from build123d import *

# Parameters (mm, degrees)
F0_W        = 50.8
F0_H        = 127
F0_R        = 50.8
F1_DEPTH    = 76.2
F2_T1_DEPTH = 76.2
F3_R        = 63.5


# Not quite as in the source:
# - a fillet or chamfer that OpenCascade refuses, or shapes differently, is made with other operations: its cross-section is extruded or revolved along the edge and cut away or added
# - a feature names something its author has since deleted; it is built from what else it names


with BuildPart() as f1:
    # F0 (on Top) → F1 (new body)
    with BuildSketch(Plane.XY):
        with BuildLine():
            Line((-3842.1031233725, -492.1847614173), (-3653.1472320591, -467.9789534788))
            ThreePointArc((-3653.1472320591, -467.9789534788), (-3683, 0), (-3653.1472320591, 467.9789534788))
            Line((-3653.1472320591, 467.9789534788), (-3842.1031233725, 492.1847614173))
            ThreePointArc((-3842.1031233725, 492.1847614173), (-3873.5, 0), (-3842.1031233725, -492.1847614173))
        make_face()
        Polygon((-3672.3184884479, -419.8900563283), (-3722.8813354916, -424.7929635108), (-3735.1386034477, -298.3858459017), (-3684.5757564041, -293.4829387192), align=None, mode=Mode.SUBTRACT)
        Polygon((-3688.3163611044, -241.9776031163), (-3739.0570382274, -244.4319227962), (-3745.1928374272, -117.5802299885), (-3694.4521603041, -115.1259103086), align=None, mode=Mode.SUBTRACT)
        with Locations((-3721.1, 0)):
            Rectangle(F0_W, F0_H, mode=Mode.SUBTRACT)
        Polygon((-3694.4521603041, 115.1259103086), (-3745.1928374272, 117.5802299885), (-3739.0570382274, 244.4319227962), (-3688.3163611044, 241.9776031163), align=None, mode=Mode.SUBTRACT)
        Polygon((-3684.5757564041, 293.4829387192), (-3735.1386034477, 298.3858459017), (-3722.8813354916, 424.7929635108), (-3672.3184884479, 419.8900563283), align=None, mode=Mode.SUBTRACT)
        with BuildLine():
            Line((-3653.1472320591, -467.9789534788), (-3275.2354494323, -419.5673376017))
            ThreePointArc((-3275.2354494323, -419.5673376016), (-3302, 0), (-3275.2354494323, 419.5673376016))
            Line((-3275.2354494323, 419.5673376017), (-3653.1472320591, 467.9789534788))
            ThreePointArc((-3653.1472320591, 467.9789534788), (-3683, 0), (-3653.1472320591, -467.9789534788))
        make_face()
        with Locations((-3492.5, 0)):
            Circle(F0_R, mode=Mode.SUBTRACT)
        with BuildLine():
            Line((-3627.8456416998, -635), (-3240.367108832, -635))
            ThreePointArc((-3240.367108832, -635), (-3259.5815655268, -527.5718128161), (-3275.2354494323, -419.5673376016))
            Line((-3275.2354494323, -419.5673376017), (-3653.1472320591, -467.9789534788))
            ThreePointArc((-3653.1472320591, -467.9789534788), (-3641.4541483351, -551.6345579938), (-3627.8456416998, -635))
        make_face()
        with BuildLine():
            Line((-3517.3268486167, -1092.2), (-3116.1359341338, -1092.2))
            ThreePointArc((-3116.1359341338, -1092.2000000001), (-3186.4620967161, -865.8309917021), (-3240.367108832, -635))
            Line((-3240.367108832, -635), (-3627.8456416998, -635))
            ThreePointArc((-3627.8456416998, -635), (-3579.8925178131, -865.3661426853), (-3517.3268486167, -1092.1999999999))
        make_face()
        with Locations((-3384.0436300379, -863.6)):
            Circle(F0_R, mode=Mode.SUBTRACT)
    extrude(amount=F1_DEPTH)

    # F2: fillet of radius 762 on 1 edges, made by hand

    # F2_s2 → F2_t1 (join)
    with BuildSketch(Plane.XY):
        with BuildLine():
            ThreePointArc((-3842.1031233725, -492.1847614173), (-3670.9916584142, -676.9720156234), (-3569.4589749529, -907.4423541626))
            Line((-3569.4589749529, -907.4423541626), (-3554.6887998841, -903.6874202833))
            ThreePointArc((-3554.6887998841, -903.6874202833), (-3603.0108161093, -686.1315301017), (-3638.030760754, -466.0424888437))
            Line((-3638.030760754, -466.0424888437), (-3655.0836966942, -452.8624821737))
            ThreePointArc((-3655.0836966942, -452.8624821737), (-3749.5616423509, -464.965386143), (-3832.7858312721, -480.1246756831))
            Line((-3832.7858312721, -480.1246756831), (-3842.1031233725, -492.1847614173))
        make_face()
    extrude(amount=F2_T1_DEPTH)

    # F3
    f3_edges = [f1.edges().sort_by_distance(p)[0] for p in [
        (-3842.103123, -492.184761, 38.1),
        (-3842.103123, 492.184761, 38.1),
        (-3275.235449, 419.567338, 38.1),
        (-3116.135934, -1092.2, 38.1),
        (-3517.326849, -1092.2, 38.1),
    ]]
    fillet(f3_edges, radius=F3_R)


solid = f1.part
Here's how the part is built. I have some questions about the finished solid (model axes, mm). A direction names the side the tool comes from. Round coordinates to 2 decimals unless told otherwise and drop trailing zeros. Loops run counter-clockwise (first coordinate to the right, second up) from the corner with the lowest first, then second, coordinate; pieces in that order, holes last.
1. We'd pull the mould along Y, two halves only. Please class faces 1 (the face through (-3153.62, -1066.79, 38.63)), 2 (the face through (-3666.08, -684.55, 37.57)), 3 (the face through (-3746.5, -1, 38)): +Y half, -Y half, draft (parallel to the pull), parting line (faces both ways), or undercut.
Answer list:
face 1: parting line
face 2: -Y half
face 3: undercut
2. If we section it at D-D on x = -3596: Write out the boundary of the cut face in (y, z).
Answer list:
outline: (-823.63, 0) - (460.66, 0) - (460.66, 76.2) - (-823.63, 76.2) - close
3. If I drill on line 1 along Y through (x, z) = (-3696.5, 34); line 2 along Y through (x, z) = (-3492.5, 42.5); line 3 along Y through (x, z) = (-3428.5, 64), over which ranges is the centre line in solid material (lowest first)?
Answer list:
line 1: y = -640.49 to -422.23, -294.64 to -242.37, -115.22 to -63.5, 63.5 to 115.22, 242.37 to 294.64, 422.23 to 473.53
line 2: y = -1088.17 to -50.8, 50.8 to 447.4
line 3: y = -1092.2 to -888.18, -839.02 to 439.2
4. If we section it at A-A on y = 0: Write out the boundary of the cut face in (x, z), plus the area to 3 significant figures.
Answer list:
outline: (-3873.5, 0) - (-3746.5, 0) - (-3746.5, 76.2) - (-3873.5, 76.2) - close; (-3695.7, 0) - (-3543.3, 0) - (-3543.3, 76.2) - (-3695.7, 76.2) - close; (-3441.7, 0) - (-3302, 0) - (-3302, 76.2) - (-3441.7, 76.2) - close
area: 31,900 mm2
5. Which directions (+Z, -Z, +X, -X, +Y, -Y) give clear straight access to the entire face, cutting with the end or side of a thin tool? Please do faces 4 (the face through (-3512, -293, 76.2)), 5 (the face through (-3709.5, 295.9, 37.6)).
Answer list:
face 4: +Z, +X, -X, +Y, -Y
face 5: +Z, -Z
6. If we section it at B-B on x = -3492.5: Write out the boundary of the cut face in (y, z), plus the area to 3 significant figures.
Answer list:
outline: (-1088.17, 0) - (-50.8, 0) - (-50.8, 76.2) - (-1088.17, 76.2) - close; (50.8, 0) - (447.4, 0) - (447.4, 76.2) - (50.8, 76.2) - close
area: 109,000 mm2
7. For P1, Ø2, axis at x = -3708, z = 9, coming from the +Y side; P2, Ø8, axis at x = -3347.5, z = 26, coming from the +Y side; P3, Ø12, axis at x = -3402.5, y = -812, coming from the -Z side; P4, Ø15, axis at x = -3722.5, z = 52, coming from the +Y side, each with a flat end and sliding along its axis, tell me the tip position at first contact or that it passes through.
Answer list:
P1: stops at y = 475.13
P2: stops at y = 429.34
P3: stops at z = 0
P4: stops at y = 477.82
8. If we section it at C-C on y = -863.6: Write out the boundary of the cut face in (x, z).
Answer list:
outline: (-3582.01, 0) - (-3434.84, 0) - (-3434.84, 76.2) - (-3582.01, 76.2) - close; (-3333.24, 0) - (-3187.07, 0) - (-3187.07, 76.2) - (-3333.24, 76.2) - close
